Design review of the part built by this model. Coordinates are the model's own, in mm. Coordinates: 2 decimals unless noted, no trailing zeros. Write each loop counter-clockwise with the first axis right and the second up, starting at its lowest first coordinate (ties: lowest second). Pieces come first, ordered by that corner, then holes. Notation, with made-up numbers: (-25, 89) -> (4, 89) arc R30 ccw to (4, 118) -> close; hole circle Ø8 at (75, 83.25). An arc over 180 degrees is marked (long way). Answer in a Markdown table with one row per item. Add a question column.
Item 1: Take a section at B-B, the plane x = -22. Write out the cut boundary in (y, z), and give its area (3 significant figures).
Item 2: To check wall thickness, follow line 1 (Y direction, x = 22, z = 2.05); line 2 (Y direction, x = 49.25, z = 0.75); line 3 (Y direction, x = -49, z = 2.1). State the ranges of each line that lie inside material, in increasing order.
Item 3: Take a section at A-A, the plane x = -49.25. Write out the cut boundary in (y, z), and give its area (3 significant figures).
Item 4: Draft analysis for pull direction Y (two halves, no side actions). For faces 1 (the face through (57.75, 0, 1)), 2 (the face through (-1, -31.5, 1)), 3 (the face through (20.5, 3.57, 1.52)), state which applies: released by +Y, released by -Y, zero draft, split by the parting line, or undercut.
Item 5: Take a section at C-C, the plane x = 49.25. Write out the cut boundary in (y, z), and give its area (3 significant figures).
from build123d import *

# Parameters (mm, degrees)
SKETCH_1_W          = 115.5
SKETCH_1_H          = 63
EXTRUDE_1_DEPTH     = 3
SKETCH_2_R          = 1.5
CUT_EXTRUDE_1_DEPTH = 66.850683368
SKETCH_3_R          = 1.5
CUT_EXTRUDE_2_DEPTH = 66.850683368


with BuildPart() as part:
    # 草图1 → 凸台-拉伸1 (new body)
    with BuildSketch(Plane.XY):
        Rectangle(SKETCH_1_W, SKETCH_1_H)
    extrude(amount=EXTRUDE_1_DEPTH)

    # 草图2 → 切除-拉伸1 (cut, through all)
    with BuildSketch(Plane.XY.offset(3)):
        with Locations((49.25, 27.5)):
            Circle(SKETCH_2_R)
        with Locations((49.25, -27.5)):
            Circle(SKETCH_2_R)
        with Locations((49.25, 15.5)):
            Circle(SKETCH_2_R)
        with Locations((49.25, -15.5)):
            Circle(SKETCH_2_R)
        with Locations((-49.25, 0)):
            Circle(SKETCH_2_R)
        with Locations((-49.25, 15)):
            Circle(SKETCH_2_R)
        with Locations((-49.25, -15)):
            Circle(SKETCH_2_R)
    extrude(amount=-CUT_EXTRUDE_1_DEPTH, mode=Mode.SUBTRACT)

    # 草图3 → 切除-拉伸2 (cut, through all)
    with BuildSketch(Plane.XY.offset(3)):
        with Locations((-22, 26.5)):
            Circle(SKETCH_3_R)
        with Locations((22, 26.5)):
            Circle(SKETCH_3_R)
        with Locations((22, 3.5)):
            Circle(SKETCH_3_R)
        with Locations((-22, 3.5)):
            Circle(SKETCH_3_R)
    extrude(amount=-CUT_EXTRUDE_2_DEPTH, mode=Mode.SUBTRACT)


solid = part.part
Answers:
| question | item | result |
|---|---|---|
| 1 | outline | (-31.5, 0) -> (2, 0) -> (2, 3) -> (-31.5, 3) -> close; (5, 0) -> (25, 0) -> (25, 3) -> (5, 3) -> close; (28, 0) -> (31.5, 0) -> (31.5, 3) -> (28, 3) -> close |
| 1 | area | 171 mm^2 |
| 2 | line 1 | y = -31.5 to 2, 5 to 25, 28 to 31.5 |
| 2 | line 2 | y = -31.5 to -29, -26 to -17, -14 to 14, 17 to 26, 29 to 31.5 |
| 2 | line 3 | y = -31.5 to -16.48, -13.52 to -1.48, 1.48 to 13.52, 16.48 to 31.5 |
| 3 | outline | (-31.5, 0) -> (-16.5, 0) -> (-16.5, 3) -> (-31.5, 3) -> close; (-13.5, 0) -> (-1.5, 0) -> (-1.5, 3) -> (-13.5, 3) -> close; (1.5, 0) -> (13.5, 0) -> (13.5, 3) -> (1.5, 3) -> close; (16.5, 0) -> (31.5, 0) -> (31.5, 3) -> (16.5, 3) -> close |
| 3 | area | 162 mm^2 |
| 4 | face 1 | zero draft |
| 4 | face 2 | released by -Y |
| 4 | face 3 | undercut |
| 5 | outline | (-31.5, 0) -> (-29, 0) -> (-29, 3) -> (-31.5, 3) -> close; (-26, 0) -> (-17, 0) -> (-17, 3) -> (-26, 3) -> close; (-14, 0) -> (14, 0) -> (14, 3) -> (-14, 3) -> close; (17, 0) -> (26, 0) -> (26, 3) -> (17, 3) -> close; (29, 0) -> (31.5, 0) -> (31.5, 3) -> (29, 3) -> close |
| 5 | area | 153 mm^2 |
